Verification items for the finished model (mm, model axes). Face numbers are marked on the shaded views. A direction names the side the tool comes from. Round coordinates to 2 decimals unless told otherwise and drop trailing zeros. Order: outer loops, then holes, each group sorted by start corner. A loop starts at its lowest first (then second) coordinate and runs counter-clockwise, first axis right, second up. Notation, with made-up numbers: M 61,-38.5 L 77,-38.5 A13 cw 77,-17.5 Z; hole C -35.5,58.25 d9. An arc over 180 degrees is marked long. Use CSV: the item, a comma, the result in double quotes. Start each with the question number.
Q1. Sectioned sample at B-B (x = 40.5). Enter the section's corners in (y, z), and give its area (3 significant figures).
Q2. Mould release check, pull along Y, two halves, no side actions. Record for the marked faces 1, 2 and 3: +Y half, -Y half, draft (parallel to the pull), parting line (faces both ways), or undercut.
Q3. Set-up check for the marked faces 4, 5 and 6: record each of +Z, -Z, +X, -X, +Y, -Y from which the full face is reachable in a straight line by a thin tool's end or side.
Q4. Scan lines: line 1 (Y direction, x = -5, z = 64.5); line 2 (X direction, y = 118.5, z = 0). Record each from-to range of solid material in increasing order.
Q5. Sectioned sample at C-C (z = -21). Enter the section's corners in (x, y).
Q6. Sectioned sample at A-A (y = 64.5). Enter the section's corners in (x, z), and give its area (3 significant figures).
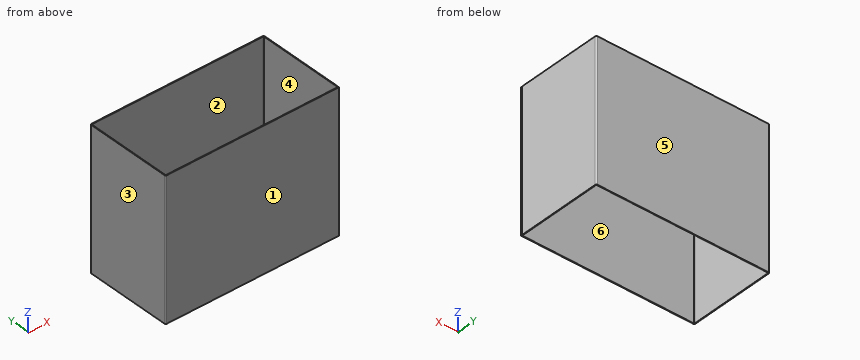
```python
from build123d import *

# Parameters (mm, degrees)
SKETCH1_W                    = 255
SKETCH1_H                    = 205
BASE_FLANGE1_DEPTH           = 1
EDGE_FLANGE1_STRIP_W         = 5.4732
EDGE_FLANGE1_STRIP_H         = 1
EDGE_FLANGE1_STRIP_CUT_DEPTH = 205
EDGE_FLANGE1_DEPTH           = 205
EDGE_FLANGE2_STRIP_W         = 5.4732
EDGE_FLANGE2_STRIP_H         = 1
EDGE_FLANGE2_STRIP_CUT_DEPTH = 205
EDGE_FLANGE2_DEPTH           = 205
EDGE_FLANGE3_STRIP_W         = 5.4732
EDGE_FLANGE3_STRIP_H         = 1
EDGE_FLANGE3_STRIP_CUT_DEPTH = 205
EDGE_FLANGE3_DEPTH           = 205


# Sheet-metal steps are written as plain solids
with BuildPart() as part:
    # Sketch1 → Base-Flange1 (new body)
    with BuildSketch(Plane(origin=(0, 0, 0), x_dir=(1, 0, 0), z_dir=(0, 1, 0))):
        Rectangle(SKETCH1_W, SKETCH1_H)
    extrude(amount=-BASE_FLANGE1_DEPTH)

    # Edge-Flange1 strip (across the edge) → Edge-Flange1 strip cut (cut)
    with BuildSketch(Plane(origin=(-127.5, 0, -102.5), x_dir=(1, 0, 0), z_dir=(0, 0, 1))):
        with Locations((-1, -0.5)):
            Rectangle(EDGE_FLANGE1_STRIP_W, EDGE_FLANGE1_STRIP_H)
    extrude(amount=EDGE_FLANGE1_STRIP_CUT_DEPTH, mode=Mode.SUBTRACT)

    # Edge-Flange1 section (across the edge) → Edge-Flange1 (add)
    with BuildSketch(Plane(origin=(-127.5, 0, -102.5), x_dir=(1, 0, 0), z_dir=(0, 0, 1))):
        with BuildLine():
            Line((0, 0.7366), (0, 127))
            Line((0, 127), (1, 127))
            Line((1, 127), (1, 0.7366))
            ThreePointArc((1, 0.7366), (1.215745145, 0.215745145), (1.7366, 0))
            Line((1.7366, 0), (1.7366, -1))
            ThreePointArc((1.7366, -1), (0.508638364, -0.491361636), (0, 0.7366))
        make_face()
    extrude(amount=EDGE_FLANGE1_DEPTH)

    # Edge-Flange2 strip (across the edge) → Edge-Flange2 strip cut (cut)
    with BuildSketch(Plane(origin=(-126.5, 127, -102.5), x_dir=(0, -1, 0), z_dir=(0, 0, 1))):
        with Locations((-1, -0.5)):
            Rectangle(EDGE_FLANGE2_STRIP_W, EDGE_FLANGE2_STRIP_H)
    extrude(amount=EDGE_FLANGE2_STRIP_CUT_DEPTH, mode=Mode.SUBTRACT)

    # Edge-Flange2 section (across the edge) → Edge-Flange2 (add)
    with BuildSketch(Plane(origin=(-126.5, 127, -102.5), x_dir=(0, -1, 0), z_dir=(0, 0, 1))):
        with BuildLine():
            Line((0, 0.7366), (0, 254))
            Line((0, 254), (1, 254))
            Line((1, 254), (1, 0.7366))
            ThreePointArc((1, 0.7366), (1.215745145, 0.215745145), (1.7366, 0))
            Line((1.7366, 0), (1.7366, -1))
            ThreePointArc((1.7366, -1), (0.508638364, -0.491361636), (0, 0.7366))
        make_face()
    extrude(amount=EDGE_FLANGE2_DEPTH)

    # Edge-Flange3 strip (across the edge) → Edge-Flange3 strip cut (cut)
    with BuildSketch(Plane(origin=(127.5, 126, -102.5), x_dir=(-1, 0, 0), z_dir=(0, 0, 1))):
        with Locations((-1, -0.5)):
            Rectangle(EDGE_FLANGE3_STRIP_W, EDGE_FLANGE3_STRIP_H)
    extrude(amount=EDGE_FLANGE3_STRIP_CUT_DEPTH, mode=Mode.SUBTRACT)

    # Edge-Flange3 section (across the edge) → Edge-Flange3 (add)
    with BuildSketch(Plane(origin=(127.5, 126, -102.5), x_dir=(-1, 0, 0), z_dir=(0, 0, 1))):
        with BuildLine():
            Line((0, 0.7366), (0, 125.5))
            Line((0, 125.5), (1, 125.5))
            Line((1, 125.5), (1, 0.7366))
            ThreePointArc((1, 0.7366), (1.215745145, 0.215745145), (1.7366, 0))
            Line((1.7366, 0), (1.7366, -1))
            ThreePointArc((1.7366, -1), (0.508638364, -0.491361636), (0, 0.7366))
        make_face()
    extrude(amount=EDGE_FLANGE3_DEPTH)


solid = part.part
```
Verdict:
1,outline,"M -1,-102.5 L 0,-102.5 L 0,102.5 L -1,102.5 Z; M 126,-102.5 L 127,-102.5 L 127,102.5 L 126,102.5 Z"
1,area,"410 mm²"
2,face 1,"-Y half"
2,face 2,"undercut"
2,face 3,"draft"
3,face 4,"+Z, -Z"
3,face 5,"+Z, -Z, +X, -X, +Y"
3,face 6,"+Z, -Z, +X"
4,line 1,"y = -1 to 0, 126 to 127"
4,line 2,"x = -127.5 to -126.5, 126.5 to 127.5"
5,outline,"M -127.5,0.74 A1.74 ccw -125.76,-1 L 127.5,-1 L 127.5,0 L -125.76,0 A0.74 cw -126.5,0.74 L -126.5,125.26 A0.74 cw -125.76,126 L 125.76,126 A0.74 cw 126.5,125.26 L 126.5,0.5 L 127.5,0.5 L 127.5,125.26 A1.74 ccw 125.76,127 L -125.76,127 A1.74 ccw -127.5,125.26 Z"
6,outline,"M -127.5,-102.5 L -126.5,-102.5 L -126.5,102.5 L -127.5,102.5 Z; M 126.5,-102.5 L 127.5,-102.5 L 127.5,102.5 L 126.5,102.5 Z"
6,area,"410 mm²"
